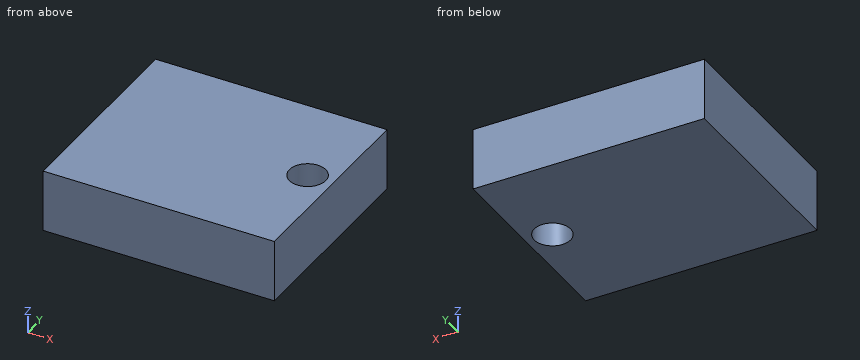
from build123d import *

# Parameters (mm, degrees)
F0_W     = 46.4574210346
F0_H     = 83.1440314651
F0_W_2   = 48.1166169047
F0_R     = 7.4407213522
F1_DEPTH = 25.4


with BuildPart() as f1:
    # F0 (on Top) → F1 (new body)
    with BuildSketch(Plane.XY):
        with Locations((-23.2287105173, -1.935724169)):
            Rectangle(F0_W, F0_H)
        with Locations((24.0583084524, -1.935724169)):
            Rectangle(F0_W_2, F0_H)
        with Locations((37.6083850861, 0)):
            Circle(F0_R, mode=Mode.SUBTRACT)
    extrude(amount=F1_DEPTH)


solid = f1.part
The model under review builds one solid part; all positions refer to its coordinate system, in mm. Coordinates: 2 decimals unless noted, no trailing zeros. Write each loop counter-clockwise with the first axis right and the second up, starting at its lowest first coordinate (ties: lowest second). Pieces come first, ordered by that corner, then holes. Notation, with made-up numbers: (16, 28) - (50, 28) arc R31 cw to (50, 54) - close; hole circle Ø7 at (-25.75, -21). An arc over 180 degrees is marked (long way). Answer as a JSON object with one key per item and string values. Group by question number.
1. Add section A-A (y = 0). Give the boundary of the cut face in (x, z).
2. Add section B-B (x = 34). Give the boundary of the cut face in (y, z), plus the area to 3 significant figures.
3. Add section C-C (z = 23.5). Give the boundary of the cut face in (x, y), plus the area to 3 significant figures.
4. To check wall thickness, follow probe 1 along Y at (x, z) = (37, 3); probe 2 along X at (y, z) = (-4.5, 2.75); probe 3 along Y at (x, z) = (32.5, 5). State the ranges of each line that lie inside material, in increasing order.
5. Clearance check with a flat-ended pin moving along its axis: pin 1 Ø9 at (x, y) = (37.61, 0) entering from +Z. State where the tip first meets the part, or that it passes through.
Findings:
{
 "1": {"outline": "(-46.46, 0) - (30.17, 0) - (30.17, 25.4) - (-46.46, 25.4) - close; (45.05, 0) - (48.12, 0) - (48.12, 25.4) - (45.05, 25.4) - close"},
 "2": {"outline": "(-43.51, 0) - (-6.51, 0) - (-6.51, 25.4) - (-43.51, 25.4) - close; (6.51, 0) - (39.64, 0) - (39.64, 25.4) - (6.51, 25.4) - close", "area": "1,780 mm²"},
 "3": {"outline": "(-46.46, -43.51) - (48.12, -43.51) - (48.12, 39.64) - (-46.46, 39.64) - close; hole circle Ø14.88 at (37.61, 0)", "area": "7,690 mm²"},
 "4": {"probe 1": "-43.51 to -7.42, 7.42 to 39.64", "probe 2": "-46.46 to 31.68, 43.53 to 48.12", "probe 3": "-43.51 to -5.41, 5.41 to 39.64"},
 "5": {"pin 1": "through"}
}
